Answer from the drawing. Dimensions are ordinates in mm from the lowest x, y and z of the part. Coordinates: 2 decimals unless noted, no trailing zeros. Write each loop counter-clockwise with the first axis right and the second up, starting at its lowest first coordinate (ties: lowest second). Pieces come first, ordered by that corner, then holes.
(1) Given pin 1 (5 mm diameter, centred on y = 20.5, z = 2.5, fed in from -X), flat-ended and moving along its own axis, determine where the tip first touches the part or whether it passes through.
(2) Section C-C on x = 0.7 is taken. Write down the section's boundary in (y, z), then the cut area to 3 significant figures.
(3) Section A-A on z = 20.5 is taken. Write down the section's boundary in (x, y).
(4) Find the intervals of material crossed by probe 1 along Z at (x, y) = (0.5, 2.5); probe 2 along Y at (x, z) = (0.35, 3.75), in increasing order.
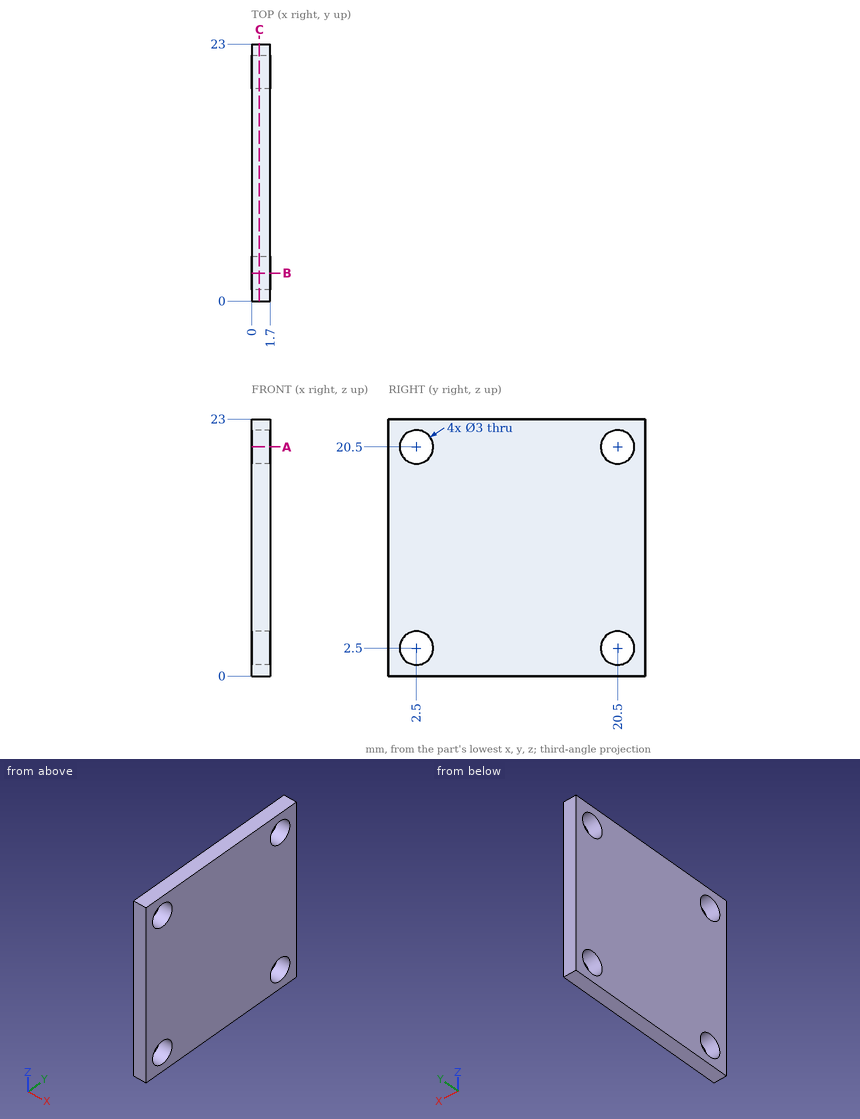
Response:
1. pin 1: stops at x = 0
2. outline: (0, 0) - (23, 0) - (23, 23) - (0, 23) - close; hole circle Ø3 at (2.5, 2.5); hole circle Ø3 at (2.5, 20.5); hole circle Ø3 at (20.5, 2.5); hole circle Ø3 at (20.5, 20.5)
2. area: 501 mm2
3. outline: (0, 0) - (1.7, 0) - (1.7, 1) - (0, 1) - close; (0, 4) - (1.7, 4) - (1.7, 19) - (0, 19) - close; (0, 22) - (1.7, 22) - (1.7, 23) - (0, 23) - close
4. probe 1: z = 0 to 1, 4 to 19, 22 to 23
4. probe 2: y = 0 to 1.67, 3.33 to 19.67, 21.33 to 23
